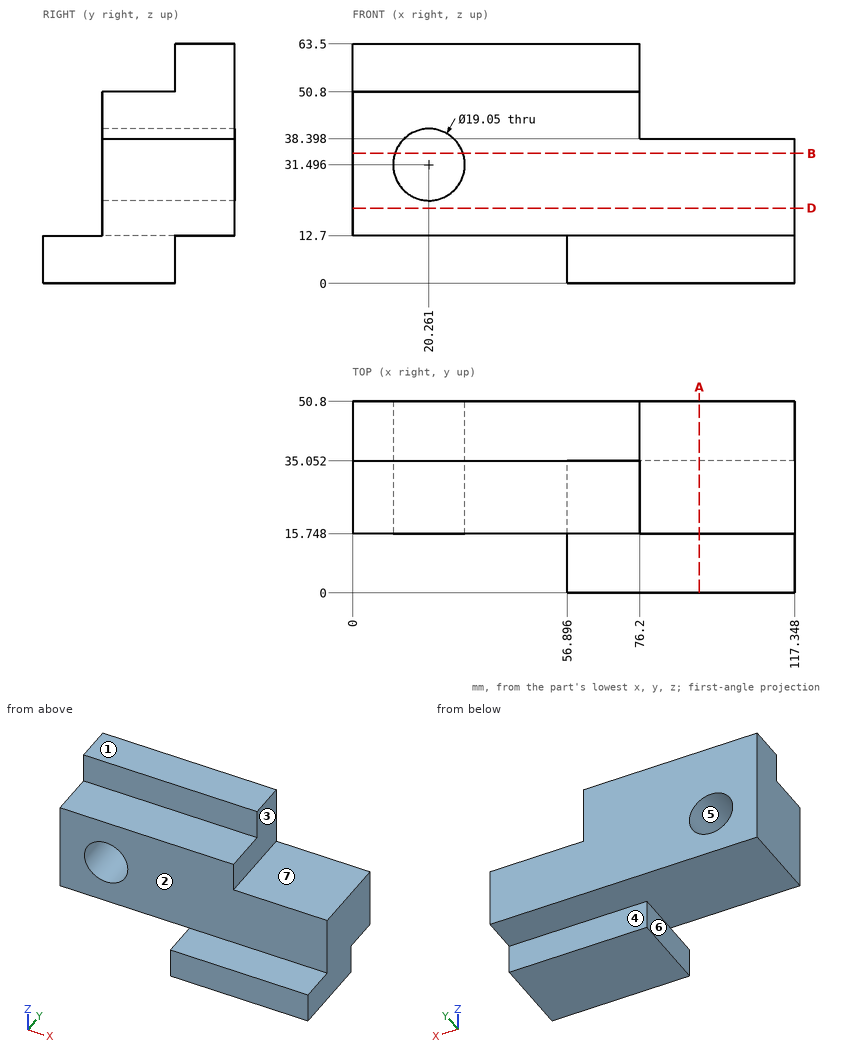
Geometry: see drawing. Coordinates: mm, zero at the bounding-box minimum. A direction names the side the tool comes from. Coordinates: 2 decimals unless noted, no trailing zeros. Write each loop counter-clockwise with the first axis right and the second up, starting at its lowest first coordinate (ties: lowest second). Pieces come first, ordered by that corner, then holes.
1) Mould query, pull axis Z, two halves, no side actions, for the marked faces 5, 6 and 7. Classes: pulls with the +Z half, pulls with the -Z half, needs draft (parallel to the pull), parting line crosses it, or undercut.
2) Section A-A on x = 92. Output: boundary loops of the cut face in (y, z).
3) Material intervals for line 1 along X through (y, z) = (42, 46.5); line 2 along Z through (x, y) = (86.5, 24.5); line 3 along Z through (x, y) = (60.5, 20.5), sorted ascending.
4) Section D-D on z = 20. Output: boundary loops of the cut face in (x, y), and give its area (3 significant figures).
5) Set-up query: the marked faces 1, 2, 3 and 4. Return all of +Z, -Z, +X, -X, +Y, -Y with unobstructed straight access to the full face (end or side cutting, diameter ignored); none if empty.
6) Pin query (flat end, axial travel): pin 1 Ø17.5 at (x, y) = (46, 38) entering from -Z; pin 2 Ø1.5 at (x, z) = (48.5, 29) entering from -Y; pin 3 Ø6 at (x, y) = (74.5, 5.5) entering from +Z. Return the tip coordinate at first contact, or that it passes through.
7) Section B-B on z = 34.5. Output: boundary loops of the cut face in (x, y), and give its area (3 significant figures).
Check result:
1. face 5: undercut
1. face 6: needs draft
1. face 7: pulls with the +Z half
2. outline: (0, 0) - (35.05, 0) - (35.05, 12.7) - (50.8, 12.7) - (50.8, 38.4) - (15.75, 38.4) - (15.75, 12.7) - (0, 12.7) - close
3. line 1: x = 0 to 76.2
3. line 2: z = 0 to 38.4
3. line 3: z = 0 to 50.8
4. outline: (0, 15.75) - (117.35, 15.75) - (117.35, 50.8) - (0, 50.8) - close
4. area: 4,110 mm2
5. face 1: +Z, +X, -X, +Y, -Y
5. face 2: +Z, +X, -X, -Y
5. face 3: +Z, +X, +Y, -Y
5. face 4: -Z, +X, -X, +Y
6. pin 1: stops at z = 12.7
6. pin 2: stops at y = 15.75
6. pin 3: stops at z = 12.7
7. outline: (0, 15.75) - (11.22, 15.75) - (11.22, 50.8) - (0, 50.8) - close; (29.3, 15.75) - (117.35, 15.75) - (117.35, 50.8) - (29.3, 50.8) - close
7. area: 3,480 mm2
